The listing builds one solid part. Answer for the finished solid, in the listing's coordinates (mm). A direction names the side the tool comes from. Round coordinates to 2 decimals unless told otherwise and drop trailing zeros. Order: outer loops, then holes, each group sorted by start corner. A loop starts at its lowest first (then second) coordinate and runs counter-clockwise, first axis right, second up. Notation, with made-up numbers: M 3,18.5 L 53,18.5 A32 ccw 53,48.5 Z; hole C 75,89 d8. An arc over 180 degrees is marked long. Write item = value, one per line. Start each with the question number.
(1) A cutting plane is placed at C-C, the plane y = 12. Determine the outline of the cut face in (x, z).
(2) Straight lines are drawn through the part: probe 1 along Y at (x, z) = (69, 11); probe 2 along Z at (x, y) = (5, -15); probe 3 along Z at (x, y) = (81.5, 3.5). For each, find the intervals that lie inside material, in ascending order. Write a range as from..to.
(3) A cutting plane is placed at A-A, the plane z = 9. Determine the outline of the cut face in (x, y).
(4) Each of these flat-tipped pins is pushed along its axis until it touches: pin 1 (0.9 mm diameter, centred on y = -19, z = 12.5, fed in from -X); pin 2 (10 mm diameter, centred on y = 1, z = -21, fed in from +X); pin 3 (1 mm diameter, centred on y = 17, z = 17.5, fed in from -X). Where does it stop, or does it pass through?
(5) A cutting plane is placed at D-D, the plane x = 46. Determine the outline of the cut face in (y, z), and give its area (3 significant figures).
(6) Which of the six approach directions +Z, -Z, +X, -X, +Y, -Y give full straight-line access (tool end or side, diameter ignored) to faces 5 (the face through (69, 19, 10)), 6 (the face through (28, -16, -10)), 7 (the face through (9, 0, 0)), 8 (the face through (94, 1.5, 16.2)), 9 (the face through (22.92, -0.22, 0.8))?
(7) A cutting plane is placed at B-B, the plane x = 87.5. Determine the outline of the cut face in (y, z).
(8) For a pull along Z with two mould halves and no side action, classify faces 1 (the face through (28, 16, -10)), 2 (the face through (46, 0, 18)), 3 (the face through (10, 0, 2)), 4 (the face through (22, 0, -1)) as released by +Z, released by -Z, zero draft, split by the parting line, or undercut.
from build123d import *

# Parameters (mm, degrees)
F1_DEPTH = 16
F2_W     = 70
F2_H     = 3
F3_DEPTH = 2
F4_W     = 50
F4_H     = 14
F5_DEPTH = 2
F6_R     = 1


with BuildPart() as f1:
    # F0 (on Front) → F1 (new body)
    with BuildSketch(Plane.XZ):
        with BuildLine():
            Line((94, 18), (0, 18))
            ThreePointArc((0, 18), (-9, 9), (0, 0))
            Line((0, 0), (19, 0))
            ThreePointArc((19, 0), (21.7681124643, -0.8361612201), (23.6103896104, -3.064978646))
            ThreePointArc((23.6103896104, -3.064978646), (50.9877645087, -35.7155080232), (92.0282848079, -47.1720964556))
            ThreePointArc((92.0282848079, -47.1720964556), (101.6638981451, -47.7394028226), (109.0104486201, -54))
            Line((109.0104486201, -54), (110.3606353849, -52.3909100723))
            ThreePointArc((110.3606353849, -52.3909100723), (102.2069764649, -45.8036465806), (91.7435184361, -45.1789545189))
            ThreePointArc((91.7435184361, -45.1789545189), (51.9754606004, -33.9725556125), (25.4545454545, -2.2909701044))
            ThreePointArc((25.4545454545, -2.2909701044), (22.87535745, 0.8293742919), (19, 2))
            Line((19, 2), (0, 2))
            ThreePointArc((0, 2), (-7, 9), (0, 16))
            Line((0, 16), (94, 16))
            Line((94, 16), (94, 18))
        make_face()
    extrude(amount=F1_DEPTH)

    # F2 (on face) → F3 (join)
    with BuildSketch(Plane.XY.offset(18)):
        with Locations((59, -17.5)):
            Rectangle(F2_W, F2_H)
    extrude(amount=-F3_DEPTH)

    # F4 (on face) → F5 (join)
    with BuildSketch(Plane.XZ.offset(19)):
        with Locations((69, 11)):
            Rectangle(F4_W, F4_H)
    extrude(amount=F5_DEPTH)

    # F6
    f6_edges = [f1.edges().sort_by_distance(p)[0] for p in [
        (69, -21, 18),
        (69, -19, 16),
    ]]
    fillet(f6_edges, radius=F6_R)

    # F7: F1 across plane


with BuildPart() as f1_1:
    add(f1.part)
    add(f1.part.mirror(Plane.XZ))


solid = f1_1.part
Reported:
q1.outline = M 0,0 L 19,0 A5 cw 23.61,-3.06 A72 ccw 92.03,-47.17 A15.18 cw 109.01,-54 L 110.36,-52.39 A17.18 ccw 91.74,-45.18 A70 cw 25.45,-2.29 A7 ccw 19,2 L 0,2 A7 cw 0,16 L 94,16 L 94,18 L 0,18 A9 ccw Z
q2.probe_1 = -21..-19, 19..21
q2.probe_2 = 0..2, 16..18
q2.probe_3 = -46.7..-44.68, 16..18
q3.outline = M -9,-16 L -7,-16 L -7,16 L -9,16 Z; M 44,-21 L 94,-21 L 94,-19 L 44,-19 Z; M 44,19 L 94,19 L 94,21 L 44,21 Z
q4.pin_1 = 44
q4.pin_2 = 41.84
q4.pin_3 = 24
q5.outline = M -21,4 L -19,4 L -19,15 A1 cw -18,16 L 18,16 A1 cw 19,15 L 19,4 L 21,4 L 21,17 A1 ccw 20,18 L -20,18 A1 ccw -21,17 Z; M -16,-32.19 L 16,-32.19 L 16,-29.64 L -16,-29.64 Z
q5.area = 214 mm²
q6.face_5 = -Z, +X, -X
q6.face_6 = -Z, -X, -Y
q6.face_7 = -Z, -X, +Y, -Y
q6.face_8 = +Z, +X, +Y, -Y
q6.face_9 = +X, +Y, -Y
q7.outline = M -21,4 L -19,4 L -19,15 A1 cw -18,16 L 18,16 A1 cw 19,15 L 19,4 L 21,4 L 21,17 A1 ccw 20,18 L -20,18 A1 ccw -21,17 Z; M -16,-47.16 L 16,-47.16 L 16,-45.16 L -16,-45.16 Z
q8.face_1 = zero draft
q8.face_2 = released by +Z
q8.face_3 = undercut
q8.face_4 = released by -Z
